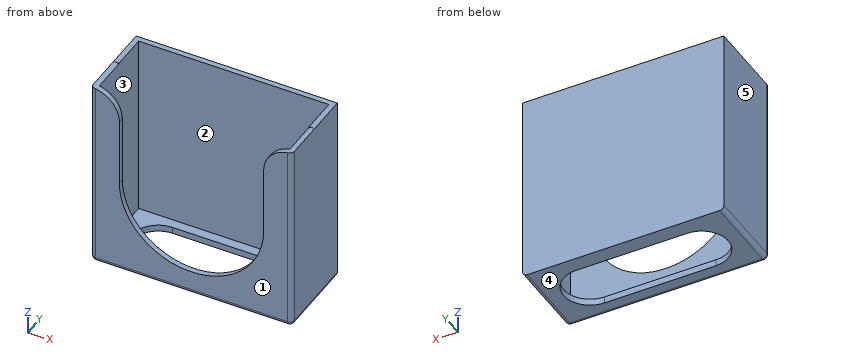
from build123d import *

# Parameters (mm, degrees)
SKETCH_W             = 46
SKETCH_H             = 19
PAD_DEPTH            = 22
POCKET_DEPTH         = 9.501
SKETCH002_W          = 43.5
SKETCH002_H          = 16.5
POCKET001_DEPTH      = 20.5
POCKET001_DEPTH_BACK = -24
POCKET002_DEPTH      = 22.001
FILLET_R             = 1


with BuildPart() as part:
    # Sketch → Pad (new body, symmetric)
    with BuildSketch(Plane.XY):
        Rectangle(SKETCH_W, SKETCH_H)
    extrude(amount=PAD_DEPTH, both=True)

    # Sketch001 → Pocket (cut, through all)
    with BuildSketch(Plane.XZ):
        with BuildLine():
            ThreePointArc((-16.5, 0), (0, -16.5), (16.5, 0))
            Line((16.5, 15.5), (16.5, 0))
            ThreePointArc((23, 22), (18.403806, 20.096194), (16.5, 15.5))
            Line((25.719499, 22), (23, 22))
            Line((25.719499, 26.595188), (25.719499, 22))
            Line((-24.273219, 26.595188), (25.719499, 26.595188))
            Line((-24.273219, 22), (-24.273219, 26.595188))
            Line((-23, 22), (-24.273219, 22))
            ThreePointArc((-16.5, 15.5), (-18.403806, 20.096194), (-23, 22))
            Line((-16.5, 15.5), (-16.5, 0))
        make_face()
    extrude(amount=POCKET_DEPTH, mode=Mode.SUBTRACT)

    # Sketch002 → Pocket001 (cut, two sides)
    with BuildSketch(Plane.XY) as pocket001_sk:
        Rectangle(SKETCH002_W, SKETCH002_H)
    extrude(amount=-POCKET001_DEPTH, mode=Mode.SUBTRACT)
    extrude(pocket001_sk.sketch, amount=-POCKET001_DEPTH_BACK, mode=Mode.SUBTRACT)

    # Sketch003 → Pocket002 (cut, through all)
    with BuildSketch(Plane.XY):
        with BuildLine():
            ThreePointArc((-12.783883, 6.033269), (-18.817152, 0), (-12.783883, -6.033269))
            Line((-12.783883, -6.033269), (12.783883, -6.033269))
            ThreePointArc((12.783883, -6.033269), (18.817152, 0), (12.783883, 6.033269))
            Line((12.783883, 6.033269), (-12.783883, 6.033269))
        make_face()
    extrude(amount=-POCKET002_DEPTH, mode=Mode.SUBTRACT)

    # Fillet
    fillet_edges = [part.edges().sort_by_distance(p)[0] for p in [
        (-23, -9.5, 0),
        (0, -9.5, -22),
        (23, -9.5, 0),
        (23, 0, -22),
        (-23, 0, -22),
    ]]
    fillet(fillet_edges, radius=FILLET_R)


solid = part.part
Geometry: final body of the model. Coordinates: model frame, mm. Face numbers are marked on the shaded views. A direction names the side the tool comes from. Give positions to 0.01 mm unless a question says otherwise; leave off trailing zeros. Loops run counter-clockwise (first coordinate to the right, second up) from the corner with the lowest first, then second, coordinate; pieces in that order, holes last. Notation, with made-up numbers: M 0.5,-1 L 10.5,-1 A31 ccw 10.5,30 Z; hole C 80.5,44 d6. An arc over 180 degrees is marked long. Put each result on its own line as item: value.
1) First-contact query: P1, Ø0.6, axis at y = -9, z = 9, coming from the +X side; P2, Ø2, axis at x = -10.5, z = 14, coming from the -Y side; P3, Ø6, axis at x = -12, y = 2, coming from the +Z side; P4, Ø5, axis at x = -6.5, y = -4, coming from the +Z side. Flat tips, straight axial feed; report the tip coordinate or a pass-through.
Computed values:
P1: stops at x = 22.98
P2: stops at y = 8.25
P3: passes through
P4: stops at z = -20.5
2) Cut plane A-A, the plane x = 0. Return the cut outline in (y, z), plus the area to 3 significant figures.
Computed values:
outline: M -9.5,-21 A1 ccw -8.5,-22 L -6.03,-22 L -6.03,-20.5 L -8.25,-20.5 L -8.25,-16.5 L -9.5,-16.5 Z; M 6.03,-22 L 9.5,-22 L 9.5,22 L 8.25,22 L 8.25,-20.5 L 6.03,-20.5 Z
area: 68.3 mm^2
3) Cut plane B-B, the plane z = 2.5. Return the cut outline in (x, y).
Computed values:
outline: M -23,-8.5 A1 ccw -22,-9.5 L -16.5,-9.5 L -16.5,-8.25 L -21.75,-8.25 L -21.75,8.25 L 21.75,8.25 L 21.75,-8.25 L 16.5,-8.25 L 16.5,-9.5 L 22,-9.5 A1 ccw 23,-8.5 L 23,9.5 L -23,9.5 Z
4) Cut plane C-C, the plane y = -3. Return the cut outline in (x, z).
Computed values:
outline: M -23,-21 A1 ccw -22,-22 L -18.02,-22 L -18.02,-20.5 L -21.75,-20.5 L -21.75,21.88 A6.5 ccw -23,22 Z; M 18.02,-22 L 22,-22 A1 ccw 23,-21 L 23,22 A6.5 ccw 21.75,21.88 L 21.75,-20.5 L 18.02,-20.5 Z
5) Material intervals for L1, parallel to X at y = -5.75, z = -5.5; L2, parallel to Y at x = -16.5, z = -6; L3, parallel to Z at x = 20.5, y = 1.75, sorted ascending. Write a range as from..to.
Computed values:
L1: x = -23..-21.75, 21.75..23
L2: y = -9.5..-8.25, 8.25..9.5
L3: z = -22..-20.5
6) Mould query, pull axis X, two halves, no side actions, for the marked faces 3, 4 and 5. Classes: released by +X, released by -X, zero draft, split by the parting line, or undercut.
Computed values:
face 3: undercut
face 4: zero draft
face 5: released by -X
7) Reachability of the marked faces 1 and 2 from +Z, -Z, +X, -X, +Y, -Y: full face, straight path, thin tool, end or side. Return the list, or none.
Computed values:
face 1: +Z, -Z, +X, -X, -Y
face 2: +Z
8) Cut plane D-D, the plane y = -7. Return the cut outline in (x, z), plus the area to 3 significant figures.
Computed values:
outline: M -23,-21 A1 ccw -22,-22 L 22,-22 A1 ccw 23,-21 L 23,22 A6.5 ccw 21.75,21.88 L 21.75,-20.5 L -21.75,-20.5 L -21.75,21.88 A6.5 ccw -23,22 Z
area: 175 mm^2
